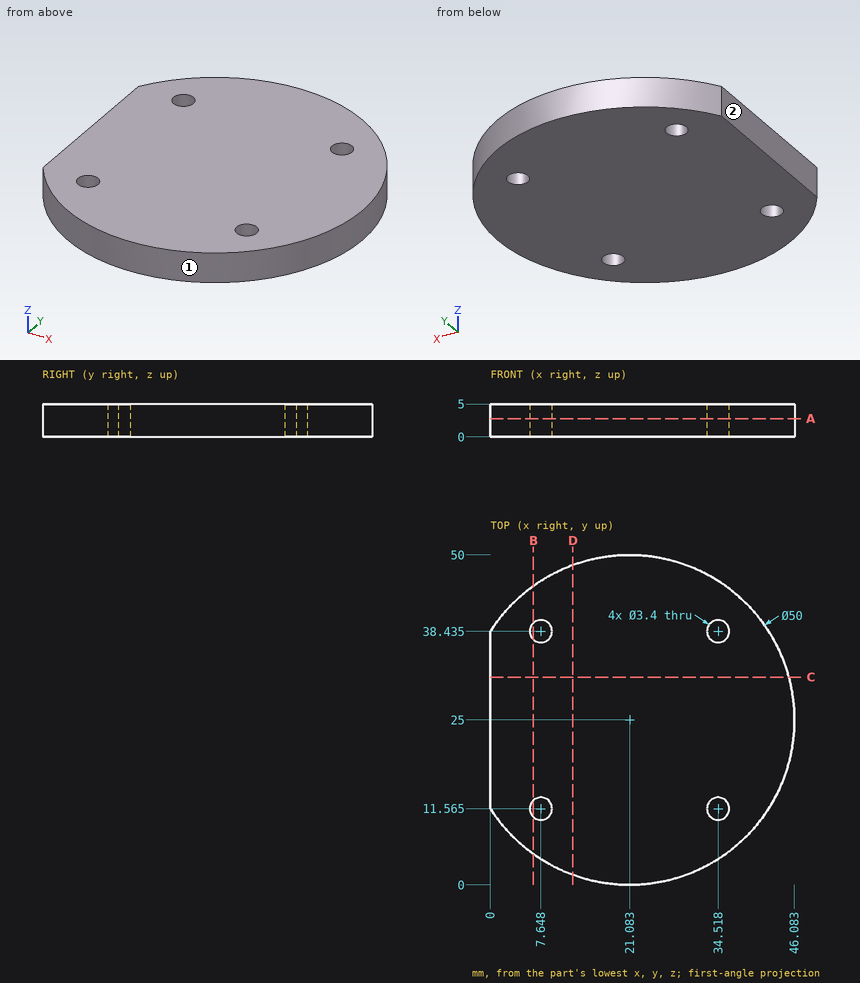
Answer from the drawing. Dimensions are ordinates in mm from the lowest x, y and z of the part. Give positions to 0.01 mm unless a question says otherwise; leave off trailing zeros. Order: outer loops, then holes, each group sorted by start corner. A loop starts at its lowest first (then second) coordinate and runs counter-clockwise, first axis right, second up. Notation, with made-up numbers: (50, 47) -> (99, 47) arc R19 cw to (99, 71) -> close; hole circle Ø3 at (29, 53). An arc over 180 degrees is marked (long way). Answer as a JSON object with one key per item and string values. Group by question number.
1. Section A-A on z = 2.8 is taken. Determine the outline of the cut face in (x, y) (1 decimal).
2. Flat-ended cylindrical pins translate along their axes: pin 1 Ø3 at (y, z) = (8.5, 4) entering from -X; pin 2 Ø2 at (x, z) = (39.5, 4) entering from +Y (1 decimal); pin 3 Ø2.5 at (x, y) = (34.52, 38.44) entering from -Z; pin 4 Ø1.5 at (x, z) = (26, 2) entering from +Y. Find the tip coordinate at first contact, or state that the pin passes through.
3. Section D-D on x = 12.5 is taken. Determine the outline of the cut face in (y, z).
4. Section C-C on y = 31.5 is taken. Determine the outline of the cut face in (x, z), plus the area to 3 significant figures.
5. Consider line 1 along X through (y, z) = (11, 2.25) (1 decimal); line 2 along Y through (x, z) = (7, 2.3) (1 decimal); line 3 along X through (y, z) = (38, 2.1) (1 decimal). Determine where each line is inside the solid, lowest interval first. Write a range as [from, to].
6. Section B-B on x = 6.5 is taken. Determine the outline of the cut face in (y, z).
7. The mould has two halves that part along Y. Classify the marked faces 1 and 2: released by +Y, released by -Y, zero draft, split by the parting line, or undercut.
Result sheet:
{
 "1": {"outline": "(0, 11.6) arc R25 ccw (long way) to (0, 38.4) -> close; hole circle Ø3.4 at (7.6, 11.6); hole circle Ø3.4 at (7.6, 38.4); hole circle Ø3.4 at (34.5, 11.6); hole circle Ø3.4 at (34.5, 38.4)"},
 "2": {"pin 1": "stops at x = 1.08", "pin 2": "stops at y = 42.9", "pin 3": "passes through", "pin 4": "stops at y = 49.65"},
 "3": {"outline": "(1.52, 0) -> (48.48, 0) -> (48.48, 5) -> (1.52, 5) -> close"},
 "4": {"outline": "(0, 0) -> (45.22, 0) -> (45.22, 5) -> (0, 5) -> close", "area": "226 mm^2"},
 "5": {"line 1": "x = [0.4, 6], [9.3, 32.9], [36.1, 41.8]", "line 2": "y = [4.3, 10], [13.1, 36.9], [40, 45.7]", "line 3": "x = [0, 6], [9.3, 32.9], [36.2, 42.4]"},
 "6": {"outline": "(4.69, 0) -> (10.31, 0) -> (10.31, 5) -> (4.69, 5) -> close; (12.82, 0) -> (37.18, 0) -> (37.18, 5) -> (12.82, 5) -> close; (39.69, 0) -> (45.31, 0) -> (45.31, 5) -> (39.69, 5) -> close"},
 "7": {"face 1": "split by the parting line", "face 2": "zero draft"}
}
